Autodesk Inventor part; units mm, degrees
ref_plane "YZ Plane" through (0, 0, 0) normal (1, 0, 0) x (0, 1, 0)
ref_plane "XZ Plane" through (0, 0, 0) normal (0, 1, 0) x (-1, 0, 0)
ref_plane "XY Plane" through (0, 0, 0) normal (0, 0, 1) x (1, 0, 0)
sketch "Base Profile" plane through (0, 0, 0) normal (0, 1, 0) x (-1, 0, 0)
  line L0 (0, 0) -> (15, 0)
  line L1 (15, 0) -> (15, -15)
  line L2 (15, -15) -> (0, -15)
  line L3 (0, -15) -> (0, 0)
  line L4 (15, 0) -> (32, 0)
  line L5 (32, 0) -> (32, -15)
  line L6 (32, -15) -> (15, -15)
  line L7 (15, -15) -> (15, 0)
  dimension "d164" = 15
  dimension "d165" = 15
  dimension "d166" = 17
  dimension "d167" = 15
extrude "Stock" add sketch "Base Profile" against normal blind 33
extrude "Extrusion Post" add sketch "Base Profile" along normal blind 15 contours L0 L1 L2 L3
sketch "Sketch27" plane through (0, -33, -15) normal (0, 0, -1) x (-1, 0, 0)
  line L0 (0, 0) -> (0, 48)
  line L1 (32, 0) -> (0, 0)
  line L2 (32, 33) -> (32, 0)
  line L3 (15, 33) -> (32, 33)
  line L4 (15, 33) -> (15, 48)
  line L5 (0, 48) -> (15, 48)
  line L6 (0, 16.5) -> (32, 16.5)
  line L7 (0, 7.5) -> (32, 7.5)
  line L8 (15, 33) -> (15, 0)
  point P0 (15, 16.5)
  point P1 (15, 7.5)
  dimension "d247" = 16.5
  dimension "d290" = 7.5
extrude "Lower Half Cut" cut sketch "Sketch27" against normal through all contours L8 L6 L2 L7
sketch "Bottom Profile" plane through (-35, -33, -15) normal (0, -1, 0) x (1, 0, 0)
  line L0 (13.5, 7.5) -> (9.5, 7.5) construction
  line L1 (13.5, 10.675) -> (9.5, 10.675)
  line L2 (9.5, 4.325) -> (13.5, 4.325)
  arc A0 (13.5, 4.325) -> (13.5, 10.675) centre (13.5, 7.5) ccw
  arc A1 (9.5, 10.675) -> (9.5, 4.325) centre (9.5, 7.5) ccw
  line L3 (3, 15) -> (3, 0)
  line L4 (35, 15) -> (3, 15)
  point P0 (11.5, 7.5)
  dimension "d291" = 4
  dimension "d292" = 6.35
  dimension "d293" = 6.5
  dimension "d294" = 7.5
extrude "Slot Cut" cut sketch "Bottom Profile" against normal blind 24
sketch "Front Hole Pattern" plane through (0, -33, 0) normal (1, 0, 0) x (0, 0, -1)
  line L0 (0, 0) -> (0, 48)
  circle A0 centre (7.5, 40.5) radius 3.175
  line L1 (0, 48) -> (15, 48)
  circle A1 centre (7.5, 21.25) radius 3.175
  line L2 (15, 0) -> (0, 0)
  dimension "d317" = 6.35
  dimension "d318" = 7.5
  dimension "d319" = 7.5
  dimension "d354" = 6.35
  dimension "d356" = 21.25
sketch "Sketch33" plane through (0, 15, 0) normal (0, 1, 0) x (1, 0, 0)
  line L0 (-15, 15) -> (-15, 0)
  line L1 (-15, 0) -> (0, 0)
  line L2 (0, 0) -> (0, 15)
  line L3 (0, 15) -> (-15, 15)
  circle A0 centre (-7.5, 7.5) radius 3.175
  dimension "d340" = 6.35
  dimension "d341" = 7.5
  dimension "d342" = 7.5
hole "Top Mounting Hole" at (-7.5, 15, -7.5) direction (0, -1, 0) diameter 3.2004 end through all counterbore diameter 6.35 counterbore depth 34.496
sketch "Rear Hole Patttern" plane through (-32, -33, -15) normal (-1, 0, 0) x (0, 0, 1)
  line L0 (15, 7.5) -> (0, 7.5)
  line L1 (0, 7.5) -> (0, 0)
  line L2 (15, 0) -> (0, 0)
  line L3 (15, 7.5) -> (15, 0)
  circle A0 centre (7.5, 2.75) radius 1.5
  line L4 (0, 16.5) -> (15, 16.5)
  line L5 (15, 33) -> (15, 16.5)
  line L6 (0, 33) -> (15, 33)
  line L7 (0, 33) -> (0, 16.5)
  circle A1 centre (7.5, 21.25) radius 1.5
  dimension "d330" = 3
  dimension "d331" = 7.5
  dimension "d352" = 3
  dimension "d358" = 2.75
  dimension "d359" = 4.75
hole "Adjustment Holes" at (-32, -30.25, -7.5) direction (1, 0, 0) diameter 2.459 depth 13.6652 tip angle 118
hole "Front Adjustment Hole" at (0, -11.75, -7.5) direction (-1, 0, 0) diameter 3.2004 end through all counterbore diameter 6.35 counterbore depth 10.675
hole "Front Mounting Hole" at (0, 7.5, -7.5) direction (-1, 0, 0) diameter 3.2004 end through all counterbore diameter 6.35 counterbore depth 10.675
fillet "Fillet2" radius 6.35 2 edges at (-32, -29.25, 0) (-32, -8.25, 0)
equation "\"d164\" = extrusionWidth"
equation "\"d165\" = extrusionWidth"
equation "\"d166\" = idlerLength"
equation "\"d167\" = d165"
equation "\"d168\" = extrusionOffset"
equation "\"extrusionWidth\" = 15"
equation "\"idlerLength\" = 17"
equation "\"bearingOffsetFromBottom\" = 7.5"
equation "\"extrusionOffset\" = 33"
equation "\"bearingStackHeight\" = 9"
equation "\"bearingSlotLength\" = 4"
equation "\"bearingClearance\" = 13"
equation "\"pinSupportLength\" = 2"
properties part number "A Idler" material "Aluminum 6061"
Can you work these out from the model? Positions are in its coordinate system, mm. A direction names the side the tool comes from. Coordinates: 2 decimals unless noted, no trailing zeros. Write each loop counter-clockwise with the first axis right and the second up, starting at its lowest first coordinate (ties: lowest second). Pieces come first, ordered by that corner, then holes. Notation, with made-up numbers: (77, 19.5) - (120, 19.5) arc R23 ccw to (120, 31.5) - close; hole circle Ø8 at (-28.75, -6.75). An arc over 180 degrees is marked (long way). Return JSON: item names as keys, results as strings.
Q1. If we section it at C-C (z = -13.5): Please give me the cut outline in (x, y), then the cut area to 3 significant figures.
Computed values:
{"outline": "(-32, -33) - (0, -33) - (0, 15) - (-15, 15) - (-15, 0) - (-32, 0) - (-32, -16.5) - (-15, -16.5) - (-15, -25.5) - (-32, -25.5) - close", "area": "1,130 mm2"}
Q2. If we section it at B-B (x = -19.5): Please give me the cut outline in (y, z), then the cut area to 3 significant figures.
Computed values:
{"outline": "(-33, -15) - (-25.5, -15) - (-25.5, -9.97) - (-33, -9.97) - close; (-33, -5.03) - (-25.5, -5.03) - (-25.5, 0) - (-33, 0) - close; (-16.5, -15) - (0, -15) - (0, 0) - (-16.5, 0) - (-16.5, -5.03) - (-9, -5.03) - (-9, -9.97) - (-16.5, -9.97) - close", "area": "286 mm2"}
Q3. On a 3-axis mill with a long thin cutter (end or side, diameter ignored), from which of +Z, -Z, +X, -X, +Y, -Y can I reach the whole of each face in a straight line? I mean faces 5 (the flat face through (-23, 0, -7)), 6 (the cylindrical face through (-18.326, -28.469, -7.57)), 7 (the flat face through (-15, -21, -8)), 8 (the cylindrical face through (-9.8, -11.727, -10.675)). Say none if no direction works.
Computed values:
{"face 5": "+Z, -Z, -X, +Y", "face 6": "-Y", "face 7": "+Z, -Z, -X", "face 8": "+X"}
Q4. If we section it at A-A (y = -16): Please give me the cut outline in (x, z) (3 decimals).
Computed values:
{"outline": "(-32, -15) - (0, -15) - (0, 0) - (-25.65, 0) arc R6.35 ccw to (-32, -6.35) - close; hole (-25.5, -10.675) - (-21.5, -10.675) arc R3.175 ccw to (-21.5, -4.325) - (-25.5, -4.325) arc R3.175 ccw to start; hole circle Ø6.35 at (-7.5, -7.5)"}
Q5. Please list where these lines run through material, in increasing order: L1, parallel to Y at x = -13.8, z = -7.5; L2, parallel to Z at x = -7.5, y = -2 (3 decimals); L3, parallel to X at y = -15, z = -7.5 (3 decimals). Write a range as from..to.
Computed values:
{"L1": "y = -33..-13.35, -10.15..5.9, 9.1..15", "L2": "z = -15..-10.675, -4.325..0", "L3": "x = -32..-28.675, -18.325..-10.675, -4.325..0"}
Q6. If we section it at D-D (y = -6): Please give me the cut outline in (x, z) (3 decimals), then the cut area to 3 significant figures.
Computed values:
{"outline": "(-32, -15) - (0, -15) - (0, 0) - (-25.65, 0) arc R6.35 ccw to (-32, -6.35) - close; hole circle Ø6.35 at (-7.5, -7.5)", "area": "440 mm2"}
Q7. I'm going to push flat-ended pins straight in: pin 1 Ø7.5 at (x, z) = (-23, -10) entering from +Y; pin 2 Ø4 at (x, z) = (-7.5, -7.5) entering from +Y; pin 3 Ø3 at (x, z) = (-26, -8.5) entering from -Y. Where does each tip first touch, or does it pass through?
Computed values:
{"pin 1": "stops at y = 0", "pin 2": "stops at y = -19.5", "pin 3": "stops at y = -9"}
Q8. Thinking about a two-plate mould opening in X: for faces 1 (the flat face through (-10, -9, 0)), 2 (the flat face through (-32, -29, -11)), 3 (the flat face through (-23, -29, -4.325)), 4 (the flat face through (-10.675, -13, -6)), which applies, +X half, -X half, draft (parallel to the pull), parting line (faces both ways), or undercut?
Computed values:
{"face 1": "draft", "face 2": "-X half", "face 3": "undercut", "face 4": "+X half"}
